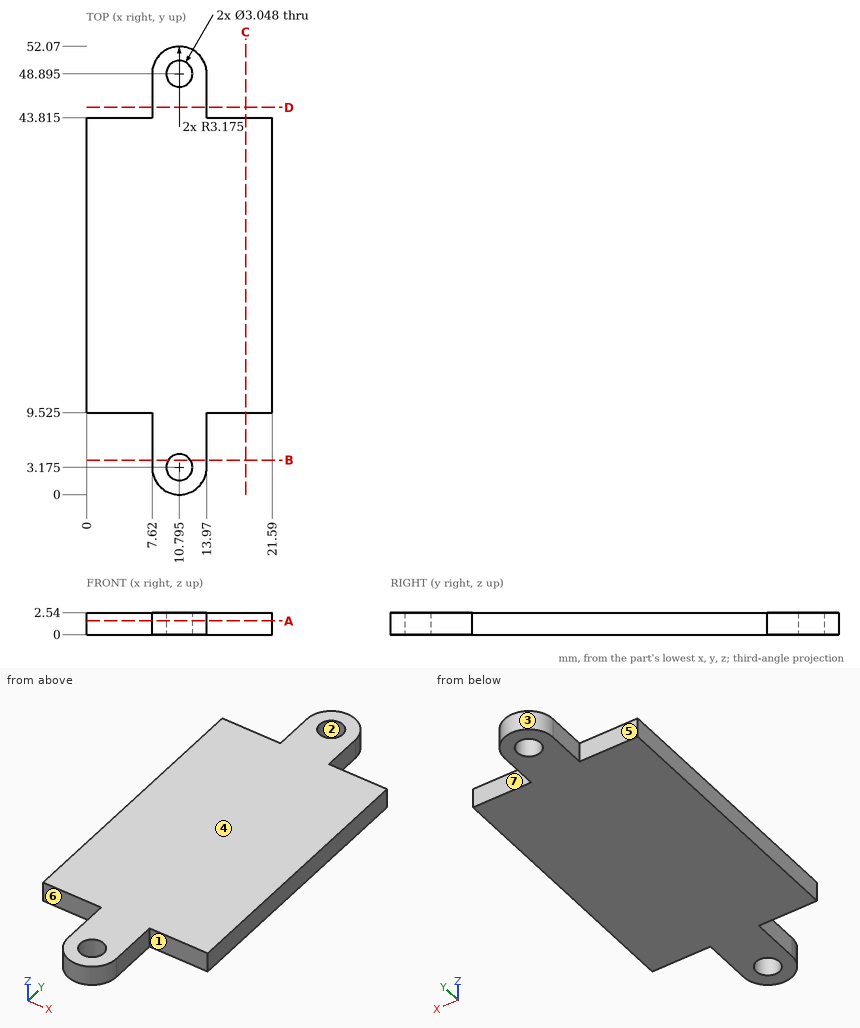
Input: dimensioned drawing with shaded views. Units: mm. Origin: part minimum x, y, z. A direction names the side the tool comes from. Coordinates: 2 decimals unless noted, no trailing zeros. Loops run counter-clockwise (first coordinate to the right, second up) from the corner with the lowest first, then second, coordinate; pieces in that order, holes last. Notation, with made-up numbers: (35, -1.5) -> (46, -1.5) arc R28 cw to (46, 18.5) -> close; hole circle Ø9 at (14, 33.25). An arc over 180 degrees is marked (long way). Use a Markdown table: item, result. Add a question column.
(1) Pin query (flat end, axial travel): pin 1 Ø1.3 at (x, z) = (4, 1) entering from -Y (3 decimals). Return the tip coordinate at first contact, or that it passes through.
(2) Section query B-B, the plane y = 4. Return loops of the section in (x, z), plus the area to 3 significant figures.
(3) Access query for the marked faces 4, 5, 6 and 7. Directions: +Z, -Z, +X, -X, +Y, -Y. A direction counts if a zero-diameter tool reaches every point of the face in a straight line with its end or side. Return the directions, or none.
(4) Section query C-C, the plane x = 18.5. Return loops of the section in (y, z) (3 decimals).
(5) Line query: line 1 along Y through (x, z) = (10.75, 1.25); line 2 along Y through (x, z) = (5.25, 1.7) (3 decimals); line 3 along Y through (x, z) = (8.75, 1.8). Output: solid intervals per line, ascending.
(6) Section query D-D, the plane y = 45. Return loops of the section in (x, z), plus the area to 3 significant figures.
(7) Mould query, pull axis X, two halves, no side actions, for the marked faces 1, 2 and 3. Classes: pulls with the +X half, pulls with the -X half, needs draft (parallel to the pull), parting line crosses it, or undercut.
(8) Section query A-A, the plane z = 1.6. Return loops of the section in (x, y) (3 decimals), plus the area to 3 significant figures.
Answer:
| question | item | result |
|---|---|---|
| 1 | pin 1 | stops at y = 9.525 |
| 2 | outline | (7.62, 0) -> (9.51, 0) -> (9.51, 2.54) -> (7.62, 2.54) -> close; (12.08, 0) -> (13.97, 0) -> (13.97, 2.54) -> (12.08, 2.54) -> close |
| 2 | area | 9.62 mm^2 |
| 3 | face 4 | +Z, +X, -X, +Y, -Y |
| 3 | face 5 | +Z, -Z, -X, +Y |
| 3 | face 6 | +Z, -Z, -X, -Y |
| 3 | face 7 | +Z, -Z, +X, +Y |
| 4 | outline | (9.525, 0) -> (43.815, 0) -> (43.815, 2.54) -> (9.525, 2.54) -> close |
| 5 | line 1 | y = 0 to 1.65, 4.7 to 47.37, 50.42 to 52.07 |
| 5 | line 2 | y = 9.525 to 43.815 |
| 5 | line 3 | y = 0.75 to 51.32 |
| 6 | outline | (7.62, 0) -> (13.97, 0) -> (13.97, 2.54) -> (7.62, 2.54) -> close |
| 6 | area | 16.1 mm^2 |
| 7 | face 1 | needs draft |
| 7 | face 2 | undercut |
| 7 | face 3 | parting line crosses it |
| 8 | outline | (0, 9.525) -> (7.62, 9.525) -> (7.62, 3.175) arc R3.175 ccw to (13.97, 3.175) -> (13.97, 9.525) -> (21.59, 9.525) -> (21.59, 43.815) -> (13.97, 43.815) -> (13.97, 48.895) arc R3.175 ccw to (7.62, 48.895) -> (7.62, 43.815) -> (0, 43.815) -> close; hole circle Ø3.048 at (10.795, 3.175); hole circle Ø3.048 at (10.795, 48.895) |
| 8 | area | 830 mm^2 |
